Here's how the part is built. I have some questions about the finished solid (model axes, mm). A direction names the side the tool comes from. Coordinates: 2 decimals unless noted, no trailing zeros. Write each loop counter-clockwise with the first axis right and the second up, starting at its lowest first coordinate (ties: lowest second). Pieces come first, ordered by that corner, then holes.
(1) For pin 1 Ø2 at (x, y) = (-4, 1) entering from +Z; pin 2 Ø4 at (y, z) = (-2.5, 3.5) entering from -X; pin 3 Ø1.5 at (x, z) = (-2, 12) entering from -Y, each with a flat end and sliding along its axis, tell me the tip position at first contact or that it passes through.
(2) Which directions (+Z, -Z, +X, -X, +Y, -Y) give clear straight access to the entire face, cutting with the end or side of a thin tool? Please do faces 1 (the flat face through (0, 0, 17.475)), 2 (the flat face through (2, -3, 5.563)).
(3) Imagine slicing it at D-D, the plane z = 16.5. List the corners of the cut face in (x, y) for me.
(4) Please list where these lines run through material, in increasing order: probe 1 along Z at (x, y) = (-0.5, 3.25); probe 2 along X at (y, z) = (1, 7.75); probe 3 along X at (y, z) = (-1.75, 3.25).
(5) Imagine slicing it at C-C, the plane z = 2.75. List the corners of the cut face in (x, y) for me.
(6) Imagine slicing it at A-A, the plane x = 0. List the corners of the cut face in (y, z) for me.
Autodesk Inventor part; units mm, degrees
ref_plane "YZ Plane" through (0, 0, 0) normal (1, 0, 0) x (0, 1, 0)
ref_plane "XZ Plane" through (0, 0, 0) normal (0, 1, 0) x (-1, 0, 0)
ref_plane "XY Plane" through (0, 0, 0) normal (0, 0, 1) x (1, 0, 0)
sketch "Sketch2" plane through (0, 0, 0) normal (0, 0, 1) x (1, 0, 0)
  circle A0 centre (0, 0) radius 5.5499
  dimension "d3" = 11.0998
extrude "Extrusion2" add sketch "Sketch2" along normal blind 5.5626
sketch "Sketch3" plane through (0, 0, 5.5626) normal (0, 0, 1) x (1, 0, 0)
  circle A0 centre (0, 0) radius 2.413
  dimension "d6" = 4.826
extrude "Extrusion3" add sketch "Sketch3" along normal blind 11.9126
chamfer "Chamfer1" distance 0.4953 angle 35 1 edges at (-2.413, 0, 17.4752) measured on face at (0.8911, -0.3521, 17.4752)
thread "Thread1"
fillet "Fillet1" radius 0.8128 1 edges at (-2.413, 0, 5.5626)
chamfer "Chamfer2" distance 0.8128 angle 45 1 edges at (-5.5499, 0, 5.5626) measured on face at (4.7214, -0.4427, 5.5626)
chamfer "Chamfer3" distance 0.8128 angle 45 1 edges at (-5.5499, 0, 0) measured on face at (1.9719, 1.8895, 0)
properties part number "13_2"
Recorded:
1. pin 1: stops at z = 5.57
1. pin 2: stops at x = -5.53
1. pin 3: stops at y = -2.06
2. face 1: +Z, +X, -X, +Y, -Y
2. face 2: +Z
3. outline: circle Ø4.83 at (0, 0)
4. probe 1: z = 0 to 5.56
4. probe 2: x = -2.2 to 2.2
4. probe 3: x = -5.27 to 5.27
5. outline: circle Ø11.1 at (0, 0)
6. outline: (-5.55, 0.81) - (-4.74, 0) - (4.74, 0) - (5.55, 0.81) - (5.55, 4.75) - (4.74, 5.56) - (3.23, 5.56) arc R0.81 cw to (2.41, 6.38) - (2.41, 17.13) - (1.92, 17.48) - (-1.92, 17.48) - (-2.41, 17.13) - (-2.41, 6.38) arc R0.81 cw to (-3.23, 5.56) - (-4.74, 5.56) - (-5.55, 4.75) - close
